For this review, take the finished solid that the model builds, in its own axes (mm). Give positions to 0.01 mm unless a question says otherwise; leave off trailing zeros. Write each loop counter-clockwise with the first axis right and the second up, starting at its lowest first coordinate (ties: lowest second). Pieces come first, ordered by that corner, then holes. Notation, with made-up numbers: M 56,29.25 L 60,29.25 A21 cw 60,49.25 Z; hole C 59.5,57.25 d6. An arc over 180 degrees is marked long. Use one line per item in the form item = value. Start each with the question number.
Q1. Consider section C-C on x = -23.5. Write out the cut boundary in (y, z).
Q2. Consider section A-A on z = 2.5. Write out the cut boundary in (x, y), and give its area (3 significant figures).
Q3. For probe 1 along X at (y, z) = (-20, 2.5); probe 2 along X at (y, z) = (-15, 1.7); probe 3 along Y at (x, z) = (4.5, 0.6), list the stretches that pass through material, from the lowest coordinate up. Write a range as [from, to].
Q4. Clearance check with flat-ended pins moving along their axes: pin 1 Ø0.9 at (y, z) = (-20.5, 1.5) entering from +X; pin 2 Ø1.5 at (y, z) = (21, 1.5) entering from -X; pin 3 Ø1.5 at (y, z) = (19.5, 0.5) entering from +X. State where each tip first meets the part, or that it passes through.
Q5. Consider section B-B on y = -7. Write out the cut boundary in (x, z).
Q6. Consider section D-D on y = 31. Write out the cut boundary in (x, z), and give its area (3 significant figures).
```python
from build123d import *

# Parameters (mm, degrees)
F0_R            = 37
F1_DEPTH        = 3
F2_DEPTH        = 3
F2_COPIES_COUNT = 6


# Not quite as in the source:
# - a pattern or mirror of a feature is missing from the dataset's text; its kind, count and spacing are read off the source's solid


with BuildPart() as f1:
    # F0 (on Top) → F1 (new body)
    with BuildSketch(Plane.XY):
        Circle(F0_R)
        with BuildLine():
            Line((1, 35.6262177595), (1, 34.9857113691))
            ThreePointArc((1, 34.9857113691), (25.099800796, 24.3926218353), (35, 0))
            ThreePointArc((35, 0), (-24.3926218353, -25.099800796), (-1, 34.9857113691))
            Line((-1, 34.9857113691), (-1, 35.6262177595))
            Line((-1, 35.6262177595), (1, 35.6262177595))
        make_face(mode=Mode.SUBTRACT)
        with BuildLine():
            ThreePointArc((-1, 34.9857113691), (0, 35), (1, 34.9857113691))
            Line((1, 34.9857113691), (1, 35.6262177595))
            Line((1, 35.6262177595), (-1, 35.6262177595))
            Line((-1, 35.6262177595), (-1, 34.9857113691))
        make_face()
    extrude(amount=F1_DEPTH)



with BuildPart() as f1b:
    # F0 (on Top) → F1, piece 2 (new body)
    with BuildSketch(Plane.XY):
        with BuildLine():
            ThreePointArc((-1, 2.2912878475), (-1.3693063938, -2.0916500663), (2.5, 0))
            ThreePointArc((2.5, 0), (2.0916500663, 1.3693063938), (1, 2.2912878475))
            Line((1, 2.2912878475), (1, 0.5877822405))
            Line((1, 0.5877822405), (-1, 0.5877822405))
            Line((-1, 0.5877822405), (-1, 2.2912878475))
        make_face()
        with BuildLine():
            Line((1, 0.5877822405), (1, 2.2912878475))
            ThreePointArc((1, 2.2912878475), (0, 2.5), (-1, 2.2912878475))
            Line((-1, 2.2912878475), (-1, 0.5877822405))
            Line((-1, 0.5877822405), (1, 0.5877822405))
        make_face()
    extrude(amount=F1_DEPTH)


with BuildPart() as f1_1:
    add(f1.part)

    add(f1b.part)  # F2 merges F1b
    # F0 (on Top) → F2 (join)
    with BuildSketch(Plane.XY):
        with BuildLine():
            Line((1, 0.5877822405), (1, 2.2912878475))
            ThreePointArc((1, 2.2912878475), (0, 2.5), (-1, 2.2912878475))
            Line((-1, 2.2912878475), (-1, 0.5877822405))
            Line((-1, 0.5877822405), (1, 0.5877822405))
        make_face()
        with BuildLine():
            ThreePointArc((-1, 2.2912878475), (0, 2.5), (1, 2.2912878475))
            Line((1, 2.2912878475), (1, 34.9857113691))
            ThreePointArc((1, 34.9857113691), (0, 35), (-1, 34.9857113691))
            Line((-1, 34.9857113691), (-1, 2.2912878475))
        make_face()
        with BuildLine():
            ThreePointArc((-1, 34.9857113691), (0, 35), (1, 34.9857113691))
            Line((1, 34.9857113691), (1, 35.6262177595))
            Line((1, 35.6262177595), (-1, 35.6262177595))
            Line((-1, 35.6262177595), (-1, 34.9857113691))
        make_face()
    f2 = extrude(amount=F2_DEPTH)

    # F2_copies: F2 ×6 about axis
    f2_copies_axis = Axis((0, 0, 0), (0, 0, 1))
    for i in range(1, F2_COPIES_COUNT):
        add(f2.rotate(f2_copies_axis, i * 360 / F2_COPIES_COUNT))


solid = f1_1.part
```
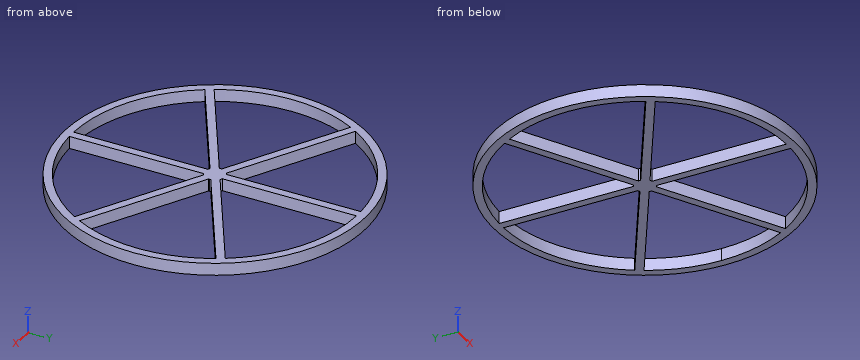
Working result:
q1.outline = M -28.58,0 L -25.94,0 L -25.94,3 L -28.58,3 Z; M -14.72,0 L -12.41,0 L -12.41,3 L -14.72,3 Z; M 12.41,0 L 14.72,0 L 14.72,3 L 12.41,3 Z; M 25.94,0 L 28.58,0 L 28.58,3 L 25.94,3 Z
q2.outline = C 0,0 d74; hole M -30.8,-16.63 L -2.48,-0.28 A2.5 cw -2.48,0.28 L -30.8,16.63 A35 ccw Z; hole M -29.8,-18.36 A35 ccw -1,-34.99 L -1,-2.29 A2.5 cw -1.48,-2.01 Z; hole M -29.8,18.36 L -1.48,2.01 A2.5 cw -1,2.29 L -1,34.99 A35 ccw Z; hole M 1,-34.99 A35 ccw 29.8,-18.36 L 1.48,-2.01 A2.5 cw 1,-2.29 Z; hole M 1,2.29 A2.5 cw 1.48,2.01 L 29.8,18.36 A35 ccw 1,34.99 Z; hole M 2.48,-0.28 L 30.8,-16.63 A35 ccw 30.8,16.63 L 2.48,0.28 A2.5 cw Z
q2.area = 863 mm²
q3.probe_1 = [-31.13, -28.72], [-1, 1], [28.72, 31.13]
q3.probe_2 = [-33.82, -31.62], [-27.98, -23.98], [-1, 1], [23.98, 27.98], [31.62, 33.82]
q3.probe_3 = [-36.73, -34.71], [-3.75, -1.44], [1.44, 3.75], [34.71, 36.73]
q4.pin_1 = 31.1
q4.pin_2 = -30.97
q4.pin_3 = 31.9
q5.outline = M -36.33,0 L -34.29,0 L -34.29,3 L -36.33,3 Z; M -14.12,0 L -10.12,0 L -10.12,3 L -14.12,3 Z; M -1,0 L 1,0 L 1,3 L -1,3 Z; M 10.12,0 L 14.12,0 L 14.12,3 L 10.12,3 Z; M 34.29,0 L 36.33,0 L 36.33,3 L 34.29,3 Z
q6.outline = M -20.2,0 L -16.25,0 L -16.25,3 L -20.2,3 Z; M -1,0 L 1,0 L 1,3 L -1,3 Z; M 16.25,0 L 20.2,0 L 20.2,3 L 16.25,3 Z
q6.area = 29.7 mm²
